```python
from build123d import *

# Parameters (mm, degrees)
F0_R      = 12.5
F0_R_2    = 7.75
F1_DEPTH  = 28
F2_W      = 3.5
F2_H      = 7.3783658981
F5_R      = 8.5
F6_DEPTH  = 5
F8_DEPTH  = 12.5
F10_DEPTH = 30


with BuildPart() as f1:
    # F0 (on Front) → F1 (new body)
    with BuildSketch(Plane.XZ):
        Circle(F0_R)
        Circle(F0_R_2, mode=Mode.SUBTRACT)
    extrude(amount=F1_DEPTH)

    # F2 (on Right) → F3 (revolve, cut)
    with BuildSketch(Plane.YZ):
        with Locations((-23.25, 6.2108170509)):
            Rectangle(F2_W, F2_H)
        with Locations((-4.75, 6.2108170509)):
            Rectangle(F2_W, F2_H)
    revolve(axis=Axis((0, -29.1106614321, 0), (0, 1, 0)), mode=Mode.SUBTRACT)

    # F5 (on mid) → F6 (join, symmetric)
    with BuildSketch(Plane.XZ.offset(14)):
        Circle(F5_R)
    extrude(amount=F6_DEPTH, both=True)

    # F7 (on Right) → F8 (cut, symmetric)
    with BuildSketch(Plane.YZ):
        with BuildLine():
            ThreePointArc((-11.9, 8), (-15.4849242405, 9.4849242405), (-14, 5.9))
            ThreePointArc((-14, 5.9), (-12.5150757595, 6.5150757595), (-11.9, 8))
        make_face()
        with BuildLine():
            ThreePointArc((-11.9, -8), (-12.5150757595, -6.5150757595), (-14, -5.9))
            ThreePointArc((-14, -5.9), (-15.4849242405, -9.4849242405), (-11.9, -8))
        make_face()
    extrude(amount=F8_DEPTH, both=True, mode=Mode.SUBTRACT)

    # F9 (on face) → F10 (cut)
    with BuildSketch(Plane.XZ.offset(28)):
        with BuildLine():
            Line((0, 12.5), (0, 7.75))
            ThreePointArc((0, 7.75), (5.4800775542, 5.4800775542), (7.75, 0))
            ThreePointArc((7.75, 0), (5.4800775542, -5.4800775542), (0, -7.75))
            Line((0, -7.75), (0, -12.5))
            ThreePointArc((0, -12.5), (8.8388347648, -8.8388347648), (12.5, 0))
            ThreePointArc((12.5, 0), (8.8388347648, 8.8388347648), (0, 12.5))
        make_face()
        with BuildLine():
            Line((0, 7.75), (0, -2.1648029558))
            Line((0, -2.1648029558), (0, -7.75))
            ThreePointArc((0, -7.75), (5.4800775542, -5.4800775542), (7.75, 0))
            ThreePointArc((7.75, 0), (5.4800775542, 5.4800775542), (0, 7.75))
        make_face()
    extrude(amount=-F10_DEPTH, mode=Mode.SUBTRACT)


solid = f1.part
```
The model under review builds one solid part; all positions refer to its coordinate system, in mm. A direction names the side the tool comes from. Give positions to 0.01 mm unless a question says otherwise; leave off trailing zeros. Write each loop counter-clockwise with the first axis right and the second up, starting at its lowest first coordinate (ties: lowest second). Pieces come first, ordered by that corner, then holes. Notation, with made-up numbers: (50.25, 20) -> (69.25, 20) arc R33 cw to (69.25, 52) -> close; hole circle Ø2 at (-33.75, -19.5). An arc over 180 degrees is marked (long way). Answer in a Markdown table with one row per item.
1) Tool access review of faces 1 (the flat face through (-8, -25, -1)), 2 (the cylindrical face through (-12.497, -13.804, 0.275)), 3 (the cylindrical face through (-7.75, -26.48, 0.17)), 4 (the cylindrical face through (-7.75, -1.48, 0.17)): name each direction out of +Z, -Z, +X, -X, +Y, -Y from which nothing blocks a thin tool from reaching the whole face with its end or side.
Worked answers:
| item | result |
|---|---|
| face 1 | +X |
| face 2 | -X, +Y, -Y |
| face 3 | +X, -Y |
| face 4 | +X, +Y |
2) Add section D-D on z = -8.75. State the section outline as (x, y) points, plus the area to 3 significant figures.
Worked answers:
| item | result |
|---|---|
| outline | (-8.93, -28) -> (0, -28) -> (0, -25) -> (-4.63, -25) -> (-4.63, -21.5) -> (0, -21.5) -> (0, -15.96) -> (-8.93, -15.96) -> close; (-8.93, -12.04) -> (0, -12.04) -> (0, -6.5) -> (-4.63, -6.5) -> (-4.63, -3) -> (0, -3) -> (0, 0) -> (-8.93, 0) -> close |
| area | 183 mm² |
3) Add section C-C on x = -3.5. Count the separate pieces of the cut face and the enclosed holes in it, plus the area to 3 significant figures.
Worked answers:
| item | result |
|---|---|
| separate pieces | 1 |
| enclosed holes | 2 |
| area | 363 mm² |
4) For L1, parallel to Y at x = -3, z = 8; L2, parallel to Y at x = -8, z = -2.25; L3, parallel to Y at x = -6.5, z = -8, list the stretches that pass through material, from the lowest coordinate up. Write a range as [from, to].
Worked answers:
| item | result |
|---|---|
| L1 | [-28, -25], [-21.5, -16.1], [-11.9, -6.5], [-3, 0] |
| L2 | [-28, -25], [-21.5, -6.5], [-3, 0] |
| L3 | [-28, -16.1], [-11.9, 0] |
5) Add section A-A on y = -12.5. State the section outline as (x, z) points, plus the area to 3 significant figures.
Worked answers:
| item | result |
|---|---|
| outline | (-10.66, -6.53) -> (0, -6.53) -> (0, 6.53) -> (-10.66, 6.53) arc R12.5 ccw to start; (-8.16, -9.47) arc R12.5 ccw to (0, -12.5) -> (0, -9.47) -> close; (-8.16, 9.47) -> (0, 9.47) -> (0, 12.5) arc R12.5 ccw to start |
| area | 189 mm² |
6) Mouldability with a two-part tool opening along Y and no side actions: class faces 5 (the flat face through (-3, -9, 0)), 6 (the cylindrical face through (-9.898, -4.726, -0.218)), 7 (the cylindrical face through (-7.75, -7.73, 0.17)) as +Y half, -Y half, draft (parallel to the pull), parting line (faces both ways), or undercut.
Worked answers:
| item | result |
|---|---|
| face 5 | +Y half |
| face 6 | undercut |
| face 7 | draft |
7) Clearance check with flat-ended pins moving along their axes: P1, Ø5, axis at y = -14, z = -8, coming from the -X side (3 decimals); P2, Ø2, axis at x = -7.5, z = 7, coming from the +Y side; P3, Ø1.5, axis at x = -10.5, y = -16, coming from the +Z side; P4, Ø2.5, axis at x = -4.5, z = -1.5, coming from the +Y side. State where each tip first meets the part, or that it passes through.
Worked answers:
| item | result |
|---|---|
| P1 | x = -11.225 |
| P2 | y = 0 |
| P3 | z = 7.82 |
| P4 | y = -9 |
8) Add section B-B on z = 0. State the section outline as (x, y) points.
Worked answers:
| item | result |
|---|---|
| outline | (-12.5, -28) -> (-7.75, -28) -> (-7.75, -25) -> (-9.9, -25) -> (-9.9, -21.5) -> (-7.75, -21.5) -> (-7.75, -19) -> (0, -19) -> (0, -9) -> (-7.75, -9) -> (-7.75, -6.5) -> (-9.9, -6.5) -> (-9.9, -3) -> (-7.75, -3) -> (-7.75, 0) -> (-12.5, 0) -> close |
